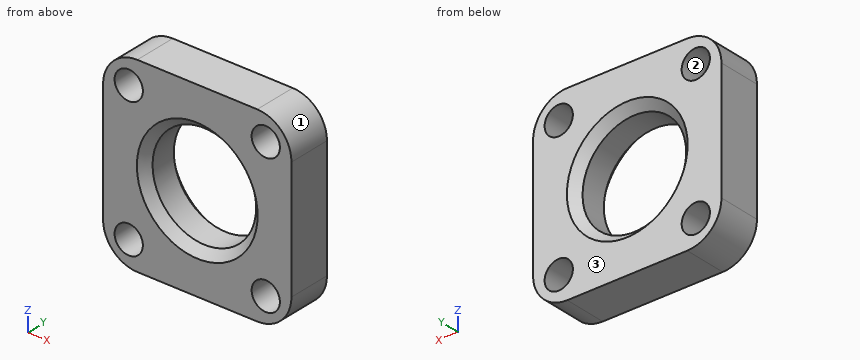
Autodesk Inventor part; units mm, degrees
ref_plane "YZ Plane" through (0, 0, 0) normal (1, 0, 0) x (0, 1, 0)
ref_plane "XZ Plane" through (0, 0, 0) normal (0, 1, 0) x (-1, 0, 0)
ref_plane "XY Plane" through (0, 0, 0) normal (0, 0, 1) x (1, 0, 0)
sketch "Sketch1" plane through (0, 0, 0) normal (0, 1, 0) x (-1, 0, 0)
  line L0 (-8, -8) -> (8, -8) construction
  line L1 (8, -8) -> (8, 8) construction
  line L2 (8, 8) -> (-8, 8) construction
  line L3 (-8, 8) -> (-8, -8) construction
  line L4 (-8, -8) -> (8, 8) construction
  line L5 (8, -8) -> (-8, 8) construction
  circle A0 centre (-8, 8) radius 1.65
  line L6 (0, 0) -> (0, 2.722) construction
  line L7 (0, 2.722) -> (0, 0) construction
  line L8 (-3.7265, 0) -> (0, 0) construction
  circle A1 centre (8, 8) radius 1.65
  line L9 (8, -8) -> (-8, -8) construction
  circle A2 centre (-8, -8) radius 1.65
  circle A3 centre (8, -8) radius 1.65
  line L10 (-11, -11) -> (11, -11)
  line L11 (11, -11) -> (11, 11)
  line L12 (11, 11) -> (-11, 11)
  line L13 (-11, 11) -> (-11, -11)
  line L14 (-11, -11) -> (11, 11) construction
  line L15 (11, -11) -> (-11, 11) construction
  circle A4 centre (0, 0) radius 6.05
  dimension "d0" = 16
  dimension "d1" = 16
  dimension "d2" = 3.3
  dimension "d3" = 22
  dimension "d4" = 22
  dimension "d5" = 12.1
extrude "Extrusion1" add sketch "Sketch1" along normal blind 5
fillet "Fillet1" radius 4 4 edges at (-11, 2.5, -11) (-11, 2.5, 11) (11, 2.5, 11) (11, 2.5, -11)
chamfer "Chamfer1" distance 1 angle 45 2 edges at (6.05, 5, 0) (6.05, 0, 0)
properties part number "Chumacera" material "ABS Plastic"
Verification items for the finished model (mm, model axes). Face numbers are marked on the shaded views. Coordinates: 2 decimals unless noted, no trailing zeros. Write each loop counter-clockwise with the first axis right and the second up, starting at its lowest first coordinate (ties: lowest second). Pieces come first, ordered by that corner, then holes. Notation, with made-up numbers: (18.25, -26.75) - (30.25, -26.75) arc R18 ccw to (30.25, -8.75) - close; hole circle Ø6 at (42, 33.5). An arc over 180 degrees is marked (long way). Write item = value, one per line.
Q1. Cross-section at C-C (x = -8). Enter the section's corners in (y, z), plus the area to 3 significant figures.
Answer:
outline = (0, -10.87) - (5, -10.87) - (5, -9.65) - (0, -9.65) - close; (0, -6.35) - (5, -6.35) - (5, 6.35) - (0, 6.35) - close; (0, 9.65) - (5, 9.65) - (5, 10.87) - (0, 10.87) - close
area = 75.7 mm²
Q2. Go/stop test with flat-tipped pins: pin 1 Ø1 at (x, z) = (5.5, 3.5) entering from -Y; pin 2 Ø4 at (x, z) = (3, -3) entering from +Y; pin 3 Ø2.5 at (x, z) = (8, -8) entering from -Y. Record where each tip stops, or that it passes through.
Answer:
pin_1 = 0.03
pin_2 = 4.19
pin_3 = through
Q3. Material ranges on L1, parallel to Z at x = 8, y = 2.15; L2, parallel to Z at x = -7, y = 4.3; L3, parallel to X at y = 1.8, z = 9, recorded low to high. Write a range as from..to.
Answer:
L1 = -10.87..-9.65, -6.35..6.35, 9.65..10.87
L2 = -11..-9.31, -6.69..6.69, 9.31..11
L3 = -10.46..-9.31, -6.69..6.69, 9.31..10.46
Q4. Cross-section at A-A (z = 0). Enter the section's corners in (x, y), plus the area to 3 significant figures.
Answer:
outline = (-11, 0) - (-7.05, 0) - (-6.05, 1) - (-6.05, 4) - (-7.05, 5) - (-11, 5) - close; (6.05, 1) - (7.05, 0) - (11, 0) - (11, 5) - (7.05, 5) - (6.05, 4) - close
area = 47.5 mm²
Q5. Mould release check, pull along Z, two halves, no side actions. Record for the marked faces 1, 2 and 3: released by +Z, released by -Z, zero draft, split by the parting line, or undercut.
Answer:
face_1 = released by +Z
face_2 = undercut
face_3 = zero draft
Q6. Cross-section at B-B (z = 8.75). Enter the section's corners in (x, y).
Answer:
outline = (-10.6, 0) - (-9.47, 0) - (-9.47, 5) - (-10.6, 5) - close; (-6.53, 0) - (6.53, 0) - (6.53, 5) - (-6.53, 5) - close; (9.47, 0) - (10.6, 0) - (10.6, 5) - (9.47, 5) - close
